Design review of the part built by this model. Coordinates are the model's own, in mm. Face numbers are marked on the shaded views. A direction names the side the tool comes from. Give positions to 0.01 mm unless a question says otherwise; leave off trailing zeros. Loops run counter-clockwise (first coordinate to the right, second up) from the corner with the lowest first, then second, coordinate; pieces in that order, holes last. Notation, with made-up numbers: (54.5, -14.75) - (70.5, -14.75) arc R12 cw to (70.5, 7.25) - close; hole circle Ø10 at (-14.75, 14.25). An arc over 180 degrees is marked (long way). Put each result on its own line as item: value. Start each with the question number.
```python
from build123d import *

# Parameters (mm, degrees)
F0_R          = 2.2
F0_W          = 5
F0_H          = 2
F1_DEPTH      = 25
F4_DEPTH      = 1.5
F4_DEPTH_BACK = 1.5
F5_R          = 1.75
F6_DEPTH      = 25


with BuildPart() as f1:
    # F0 (on Top) → F1 (new body)
    with BuildSketch(Plane.XY):
        with BuildLine():
            Line((-48.139875, 23.066107), (-47.886185, 22.919639))
            ThreePointArc((-47.886185, 22.919639), (-47.881315, 23.026134), (-47.879692, 23.132728))
            ThreePointArc((-47.879692, 23.132728), (-54.494673, 24.728627), (-49.33506, 20.292046))
            Line((-49.33506, 20.292046), (-49.639875, 20.468031))
            Line((-49.639875, 20.468031), (-48.139875, 23.066107))
        make_face()
        with Locations((-51.379692, 23.132728)):
            Circle(F0_R, mode=Mode.SUBTRACT)
        with BuildLine():
            ThreePointArc((-49.33506, 20.292046), (-48.31476, 21.442701), (-47.886185, 22.919639))
            Line((-47.886185, 22.919639), (-48.139875, 23.066107))
            Line((-48.139875, 23.066107), (-49.639875, 20.468031))
            Line((-49.639875, 20.468031), (-49.33506, 20.292046))
        make_face()
        with BuildLine():
            Line((-23.659113, 5.468031), (-23.659113, 8.468031))
            Line((-23.659113, 8.468031), (-22.855266, 8.468031))
            Line((-22.855266, 8.468031), (-47.886185, 22.919639))
            ThreePointArc((-47.886185, 22.919639), (-48.31476, 21.442701), (-49.33506, 20.292046))
            Line((-49.33506, 20.292046), (-23.659113, 5.468031))
        make_face()
        with Locations((-13.659113, 4.468031)):
            Rectangle(F0_W, F0_H)
        Polygon((-3.659113, 8.468031), (-22.855266, 8.468031), (-22.159113, 8.066107), (-23.659113, 5.468031), (-16.159113, 5.468031), (-11.159113, 5.468031), (-3.659113, 5.468031), align=None)
        Polygon((-22.855266, 8.468031), (-23.659113, 8.468031), (-23.659113, 5.468031), (-22.159113, 8.066107), align=None)
    extrude(amount=F1_DEPTH)

    # F3 (on offset) → F4 (join, two sides)
    with BuildSketch(Plane.XY.offset(12.5)) as f4_sk:
        Polygon((-3.659113, 8.468031), (-47.886185, 22.919639), (-22.855266, 8.468031), align=None)
    extrude(amount=F4_DEPTH)
    extrude(f4_sk.sketch, amount=-F4_DEPTH_BACK)

    # F5 (on face) → F6 (cut)
    with BuildSketch(Plane(origin=(0, 8.468031, 0), x_dir=(-1, 0, 0), z_dir=(0, 1, 0))):
        with Locations((13.659113, 3.913301)):
            Circle(F5_R)
        with Locations((13.659113, 21.086699)):
            Circle(F5_R)
    extrude(amount=-F6_DEPTH, mode=Mode.SUBTRACT)


solid = f1.part
```
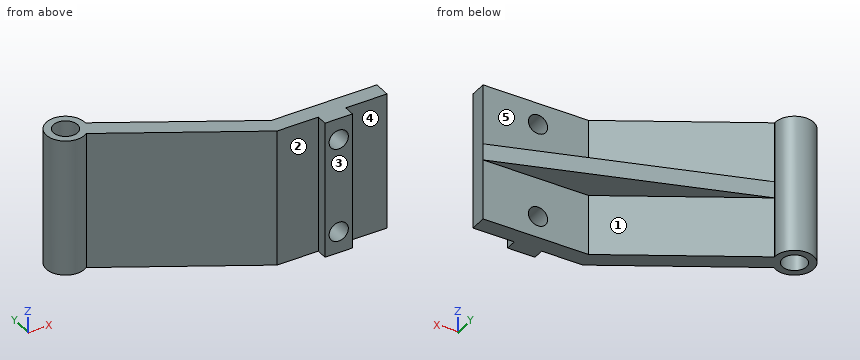
Item 1: Consider section A-A (z = 17.5). State the section outline as (x, y) points.
Item 2: Consider section D-D (x = -36). State the section outline as (y, z) points.
Item 3: Consider section B-B (z = 22.25). State the section outline as (x, y) points, plus the area to 3 significant figures.
Item 4: For L1, parallel to X at y = 23, z = 6; L2, parallel to Z at x = -22, y = 12.25; L3, parallel to Y at x = -14, z = 18, list the stretches that pass through material, from the lowest coordinate up. Write a range as from..to.
Item 5: For P1, Ø7, axis at x = -27, y = 13.5, coming from the -Z side; P2, Ø12, axis at y = 6, z = 21, coming from the -X side; P3, Ø3.5, axis at x = -15, z = 5.5, coming from the +Y side; P4, Ø8.5, axis at x = -21, z = 9.5, coming from the -Y side, all flat-tipped, find the tip position at first contact; note any pin that passes through.
Item 6: Consider section C-C (y = 11). State the section outline as (x, z) points.
Item 7: Machinability: for the marked faces 1, 2, 3, 4 and 5, which of the approach directions +Z, -Z, +X, -X, +Y, -Y give a long, thin tool a straight path to every point of the face, cutting with its end or side? Answer none if there is none.
Geometry says:
1. outline: (-49.34, 20.29) - (-23.66, 5.47) - (-16.16, 5.47) - (-16.16, 3.47) - (-11.16, 3.47) - (-11.16, 5.47) - (-3.66, 5.47) - (-3.66, 8.47) - (-22.86, 8.47) - (-47.89, 22.92) arc R3.5 ccw to (-47.88, 23.13) arc R3.5 ccw (long way) to start; hole circle Ø4.4 at (-51.38, 23.13)
2. outline: (12.59, 0) - (16.06, 0) - (16.06, 11) - (19.04, 11) - (19.04, 14) - (16.06, 14) - (16.06, 25) - (12.59, 25) - close
3. outline: (-49.34, 20.29) - (-23.66, 5.47) - (-16.16, 5.47) - (-16.16, 3.47) - (-14.97, 3.47) - (-14.97, 8.47) - (-22.86, 8.47) - (-47.89, 22.92) arc R3.5 ccw to (-47.88, 23.13) arc R3.5 ccw (long way) to start; (-12.35, 3.47) - (-11.16, 3.47) - (-11.16, 5.47) - (-3.66, 5.47) - (-3.66, 8.47) - (-12.35, 8.47) - close; hole circle Ø4.4 at (-51.38, 23.13)
3. area: 166 mm2
4. L1: x = -54.88..-53.58, -49.18..-47.88
4. L2: z = 11..14
4. L3: y = 3.47..8.47
5. P1: stops at z = 0
5. P2: stops at x = -34.97
5. P3: stops at y = 8.47
5. P4: stops at y = 5.47
6. outline: (-33.24, 0) - (-27.24, 0) - (-27.24, 11) - (-11.41, 11) - (-11.41, 14) - (-27.24, 14) - (-27.24, 25) - (-33.24, 25) - close
7. face 1: -Z, +X, +Y
7. face 2: +Z, -Z, -X, -Y
7. face 3: +Z, -Z, +X, -X, -Y
7. face 4: +Z, -Z, +X, -Y
7. face 5: +Z, +X, +Y
